```python
from build123d import *

# Parameters (mm, degrees)
SKETCH1_R           = 10
SKETCH1_R_2         = 1.05
SKETCH1_R_3         = 4
BOSS_EXTRUDE1_DEPTH = 4
SKETCH2_R           = 7.5
CUT_EXTRUDE1_DEPTH  = 10
BOSS_EXTRUDE2_START = -4
SKETCH3_R           = 4
BOSS_EXTRUDE2_DEPTH = 4


with BuildPart() as part:
    # Sketch1 → Boss-Extrude1 (new body)
    with BuildSketch(Plane.XY):
        Circle(SKETCH1_R)
        with Locations((-7, 0)):
            Circle(SKETCH1_R_2, mode=Mode.SUBTRACT)
        with Locations((0, 7)):
            Circle(SKETCH1_R_2, mode=Mode.SUBTRACT)
        with Locations((7, 0)):
            Circle(SKETCH1_R_2, mode=Mode.SUBTRACT)
        with Locations((4.949747468, 4.949747468)):
            Circle(SKETCH1_R_2, mode=Mode.SUBTRACT)
        with Locations((4.949747468, -4.949747468)):
            Circle(SKETCH1_R_2, mode=Mode.SUBTRACT)
        with Locations((0, -7)):
            Circle(SKETCH1_R_2, mode=Mode.SUBTRACT)
        with Locations((-4.949747468, -4.949747468)):
            Circle(SKETCH1_R_2, mode=Mode.SUBTRACT)
        with Locations((-4.949747468, 4.949747468)):
            Circle(SKETCH1_R_2, mode=Mode.SUBTRACT)
        Circle(SKETCH1_R_3, mode=Mode.SUBTRACT)
    extrude(amount=-BOSS_EXTRUDE1_DEPTH)

    # Sketch2 → Cut-Extrude1 (cut)
    with BuildSketch(Plane(origin=(0, 0, -4), x_dir=(-1, 0, 0), z_dir=(0, 0, -1))):
        with Locations((0, -12.82)):
            Circle(SKETCH2_R)
    extrude(amount=-CUT_EXTRUDE1_DEPTH, mode=Mode.SUBTRACT)

    # Sketch3 → Boss-Extrude2 (add)
    with BuildSketch(Plane(origin=(0, 0, -4), x_dir=(-1, 0, 0), z_dir=(0, 0, -1)).offset(BOSS_EXTRUDE2_START)):
        Circle(SKETCH3_R)
    extrude(amount=BOSS_EXTRUDE2_DEPTH)


solid = part.part
```
Can you work these out from the model? Positions are in its coordinate system, mm. Round coordinates to 2 decimals unless told otherwise and drop trailing zeros. Order: outer loops, then holes, each group sorted by start corner. A loop starts at its lowest first (then second) coordinate and runs counter-clockwise, first axis right, second up. Notation, with made-up numbers: (-12.5, 45) -> (8.5, 45) arc R24 cw to (8.5, 68) -> close; hole circle Ø7 at (-30.75, 61.25). An arc over 180 degrees is marked (long way). Return JSON: item names as keys, results as strings. Group by question number.
1. I need wall thicknesses on line 1 (Y direction, x = 4.5, z = -2.35); line 2 (Y direction, x = -4.25, z = -1.05); line 3 (X direction, y = 5, z = -2.05). Which ranges of each line are inside material? Lowest first, please. Write a range as [from, to].
2. We'd pull the mould along X, two halves only. Please class faces 1 (the face through (-1.05, 7.05, -1.97)), 2 (the face through (0, 10, -2)), 3 (the face through (0, 1, -4)): released by +X, released by -X, zero draft, split by the parting line, or undercut.
3. If we section it at C-C, the plane z = -3.45: Write out the boundary of the cut face in (x, y), then the cut area to 3 significant figures.
4. If we section it at A-A, the plane y = 0: Write out the boundary of the cut face in (x, z), then the cut area to 3 significant figures.
5. If we section it at B-B, the plane x = -7: Write out the boundary of the cut face in (y, z).
6. Will these pins go through, and if not, where does the flat tip stop? pin 1 (1 mm diameter, centred on x = -4, z = -3, fed in from +Y); pin 2 (2 mm diameter, centred on x = -5.5, z = -1.5, fed in from -Y); pin 3 (1.5 mm diameter, centred on x = 3.5, z = -1, fed in from +Y).
Output values:
{
 "1": {"line 1": "[-6.82, -5.9], [-4, 4], [5.9, 8.93]", "line 2": "[-6.64, -5.73], [-4.17, 4.17], [5.73, 9.05]", "line 3": "[-8.66, -6], [-3.9, 3.9], [6, 8.66]"},
 "2": {"face 1": "undercut", "face 2": "split by the parting line", "face 3": "zero draft"},
 "3": {"outline": "(-5.84, -8.12) arc R7.5 cw to (5.84, -8.12) arc R10 ccw (long way) to start; hole circle Ø2.1 at (-7, 0); hole circle Ø2.1 at (-4.95, -4.95); hole circle Ø2.1 at (-4.95, 4.95); hole circle Ø2.1 at (0, 7); hole circle Ø2.1 at (4.95, -4.95); hole circle Ø2.1 at (4.95, 4.95); hole circle Ø2.1 at (7, 0)", "area": "252 mm²"},
 "4": {"outline": "(-10, -4) -> (-8.05, -4) -> (-8.05, 0) -> (-10, 0) -> close; (-5.95, -4) -> (5.95, -4) -> (5.95, 0) -> (-5.95, 0) -> close; (8.05, -4) -> (10, -4) -> (10, 0) -> (8.05, 0) -> close", "area": "63.2 mm²"},
 "5": {"outline": "(-7.14, -4) -> (-1.05, -4) -> (-1.05, 0) -> (-7.14, 0) -> close; (1.05, -4) -> (7.14, -4) -> (7.14, 0) -> (1.05, 0) -> close"},
 "6": {"pin 1": "y = 9.37", "pin 2": "y = -8.12", "pin 3": "y = 9.61"}
}
